from build123d import *

# Parameters (mm, degrees)
PAD_DEPTH    = 90
THICKNESS_T  = -1.4
SKETCH001_W  = 1.4
SKETCH001_H  = 76.2
PAD001_DEPTH = 88.6


with BuildPart() as part:
    # Sketch → Pad (new body)
    with BuildSketch(Plane.XY):
        with BuildLine():
            Line((-98, 39.5), (98, 39.5))
            ThreePointArc((100, 37.5), (99.414214, 38.914214), (98, 39.5))
            Line((100, 37.5), (100, -37.5))
            ThreePointArc((98, -39.5), (99.414214, -38.914214), (100, -37.5))
            Line((98, -39.5), (-98, -39.5))
            ThreePointArc((-100, -37.5), (-99.414214, -38.914214), (-98, -39.5))
            Line((-100, -37.5), (-100, 37.5))
            ThreePointArc((-98, 39.5), (-99.414214, 38.914214), (-100, 37.5))
        make_face()
    extrude(amount=PAD_DEPTH)

    # Thickness
    thickness_openings = [part.faces().sort_by_distance(p)[0] for p in [
        (0, 0, 90),
    ]]
    offset(amount=THICKNESS_T, openings=thickness_openings)

    # Sketch001 (on Face19 of Thickness) → Pad001 (join)
    with BuildSketch(Plane.XY.offset(1.4)):
        with Locations((-33.966667, 0)):
            Rectangle(SKETCH001_W, SKETCH001_H)
        with Locations((33.969422, 0)):
            Rectangle(SKETCH001_W, SKETCH001_H)
    extrude(amount=PAD001_DEPTH)


solid = part.part
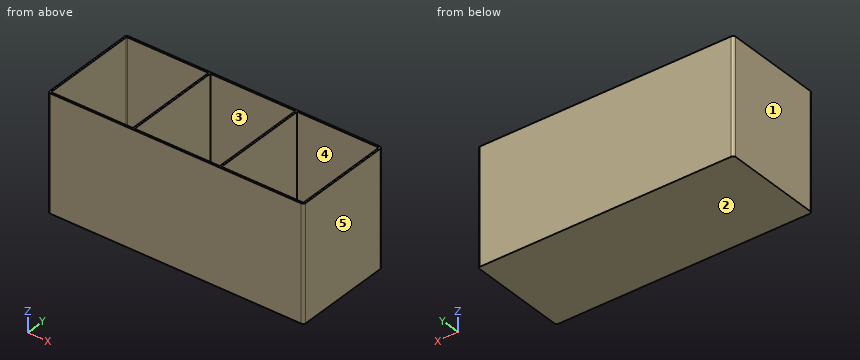
Geometry: final body of the model. Coordinates: model frame, mm. Face numbers are marked on the shaded views. A direction names the side the tool comes from. Coordinates: 2 decimals unless noted, no trailing zeros. Order: outer loops, then holes, each group sorted by start corner. A loop starts at its lowest first (then second) coordinate and runs counter-clockwise, first axis right, second up.
(1) Material intervals for probe 1 along X at (y, z) = (18, 40); probe 2 along Y at (x, z) = (83.5, 51); probe 3 along Z at (x, y) = (54, -36), sorted ascending.
(2) Section query B-B (z = 35). Return the cut outline in (x, y), plus the area to 3 significant figures.
(3) Access query for the marked faces 4 and 5. Directions: +Z, -Z, +X, -X, +Y, -Y. A direction counts if a zero-diameter tool reaches every point of the face in a straight line with its end or side. Return the directions, or none.
(4) Section query C-C (x = -26.5). Return the cut outline in (y, z).
(5) Draft query along X for the marked faces 1, 2 and 3. Return one class per face: pulls with the +X half, pulls with the -X half, needs draft (parallel to the pull), parting line crosses it, or undercut.
(6) Section query A-A (y = 4). Return the cut outline in (x, z), plus the area to 3 significant figures.
(7) First-contact query: pin 1 (2 mm diameter, centred on x = -41, y = -22, fed in from +Z). Flat tip, straight axial feed; report the tip coordinate or a pass-through.
Solution:
1. probe 1: x = -100 to -98.6, -34.67 to -33.27, 33.27 to 34.67, 98.6 to 100
1. probe 2: y = -39.5 to -38.1, 38.1 to 39.5
1. probe 3: z = 0 to 1.4
2. outline: (-100, -37.5) arc R2 ccw to (-98, -39.5) - (98, -39.5) arc R2 ccw to (100, -37.5) - (100, 37.5) arc R2 ccw to (98, 39.5) - (-98, 39.5) arc R2 ccw to (-100, 37.5) - close; hole (-98.6, -37.5) arc R0.6 ccw to (-98, -38.1) - (-34.67, -38.1) - (-34.67, 38.1) - (-98, 38.1) arc R0.6 ccw to (-98.6, 37.5) - close; hole (-33.27, -38.1) - (33.27, -38.1) - (33.27, 38.1) - (-33.27, 38.1) - close; hole (34.67, -38.1) - (98, -38.1) arc R0.6 ccw to (98.6, -37.5) - (98.6, 37.5) arc R0.6 ccw to (98, 38.1) - (34.67, 38.1) - close
2. area: 984 mm2
3. face 4: +Z
3. face 5: +Z, -Z, +X, +Y, -Y
4. outline: (-39.5, 0) - (39.5, 0) - (39.5, 90) - (38.1, 90) - (38.1, 1.4) - (-38.1, 1.4) - (-38.1, 90) - (-39.5, 90) - close
5. face 1: pulls with the -X half
5. face 2: needs draft
5. face 3: undercut
6. outline: (-100, 0) - (100, 0) - (100, 90) - (98.6, 90) - (98.6, 1.4) - (34.67, 1.4) - (34.67, 90) - (33.27, 90) - (33.27, 1.4) - (-33.27, 1.4) - (-33.27, 90) - (-34.67, 90) - (-34.67, 1.4) - (-98.6, 1.4) - (-98.6, 90) - (-100, 90) - close
6. area: 776 mm2
7. pin 1: stops at z = 1.4
